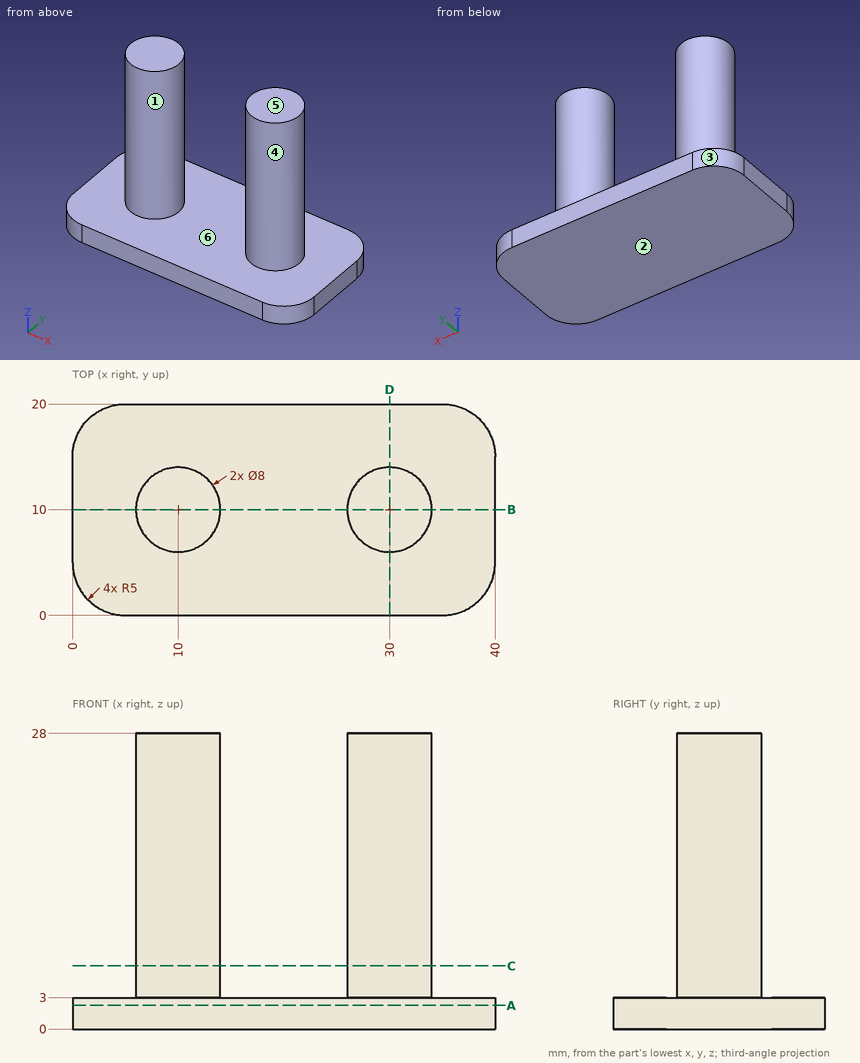
Part print with two shaded views. Sizes in mm from the minimum x, y, z corner. A direction names the side the tool comes from. Round coordinates to 2 decimals unless told otherwise and drop trailing zeros. Write each loop counter-clockwise with the first axis right and the second up, starting at its lowest first coordinate (ties: lowest second). Pieces come first, ordered by that corner, then holes. Notation, with made-up numbers: (-19, 67.25) - (27, 67.25) arc R32 cw to (27, 100.25) - close; hole circle Ø8 at (-18.75, 41). An arc over 180 degrees is marked (long way). Use CSV: the item, a comma, the result in double quotes.
Item 1: Slice it at D-D, the plane x = 30. Write the cut outline in (y, z), then the cut area to 3 significant figures.
Results list:
outline,"(0, 0) - (20, 0) - (20, 3) - (14, 3) - (14, 28) - (6, 28) - (6, 3) - (0, 3) - close"
area,"260 mm²"
Item 2: Slice it at B-B, the plane y = 10. Write the cut outline in (x, z), then the cut area to 3 significant figures.
Results list:
outline,"(0, 0) - (40, 0) - (40, 3) - (34, 3) - (34, 28) - (26, 28) - (26, 3) - (14, 3) - (14, 28) - (6, 28) - (6, 3) - (0, 3) - close"
area,"520 mm²"
Item 3: Pull direction X, two halves, no side cores. Call the marked faces 3, 4, 5 and 6: pulls with the +X half, pulls with the -X half, needs draft (parallel to the pull), parting line crosses it, or undercut.
Results list:
face 3,"pulls with the -X half"
face 4,"undercut"
face 5,"needs draft"
face 6,"undercut"
Item 4: Tool access for the marked faces 1 and 2: list every direction of +Z, -Z, +X, -X, +Y, -Y with a clear straight run to the whole face (end or side of a thin tool).
Results list:
face 1,"+Z"
face 2,"-Z, +X, -X, +Y, -Y"
Item 5: Slice it at A-A, the plane z = 2.25. Write the cut outline in (x, y).
Results list:
outline,"(0, 5) arc R5 ccw to (5, 0) - (35, 0) arc R5 ccw to (40, 5) - (40, 15) arc R5 ccw to (35, 20) - (5, 20) arc R5 ccw to (0, 15) - close"
Item 6: Flat gauge pins, fed straight in: P1, Ø10, axis at x = 23.5, y = 5.5, coming from the +Z side; P2, Ø5, axis at y = 12.5, z = 16.5, coming from the -X side; P3, Ø4, axis at x = 13.5, y = 16.5, coming from the +Z side; P4, Ø5, axis at y = 7, z = 20.5, coming from the +X side. Where does each tip first touch, or does it go through?
Results list:
P1,"stops at z = 28"
P2,"stops at x = 6"
P3,"stops at z = 3"
P4,"stops at x = 33.97"
Item 7: Wall check: L1, parallel to Z at x = 17.5, y = 3; L2, parallel to X at y = 7.25, z = 21.75; L3, parallel to X at y = 13.5, z = 15.5. Give the ranges that are in metal, low to high.
Results list:
L1,"z = 0 to 3"
L2,"x = 7.1 to 12.9, 27.1 to 32.9"
L3,"x = 8.06 to 11.94, 28.06 to 31.94"
Item 8: Slice it at C-C, the plane z = 6. Write the cut outline in (x, y), then the cut area to 3 significant figures.
Results list:
outline,"circle Ø8 at (10, 10); circle Ø8 at (30, 10)"
area,"101 mm²"
